Could you check a few things on this model? Use its own coordinates, in mm. A direction names the side the tool comes from. Give positions to 0.01 mm unless a question says otherwise; leave off trailing zeros. Write each loop counter-clockwise with the first axis right and the second up, starting at its lowest first coordinate (ties: lowest second). Pieces come first, ordered by that corner, then holes. Notation, with made-up numbers: M 26.25,23 L 69.25,23 A16 ccw 69.25,41 Z; hole C -26.75,55 d1. An arc over 180 degrees is marked long. Answer as CSV lines item,"result". Start each with the question number.
from build123d import *

# Parameters (mm, degrees)
F0_R     = 1.55
F1_DEPTH = 6


with BuildPart() as f1:
    # F0 (on Top) → F1 (new body)
    with BuildSketch(Plane.XY):
        Polygon((-284.438, 0), (0, 0), (0, 40.6), (-6, 40.6), (-6, 55.6), (0, 55.6), (0, 100.6), (-6, 100.6), (-6, 115.6), (0, 115.6), (0, 156.2), (-284.438, 156.2), (-284.438, 115.6), (-278.438, 115.6), (-278.438, 100.6), (-284.438, 100.6), (-284.438, 55.6), (-278.438, 55.6), (-278.438, 40.6), (-284.438, 40.6), align=None)
        with Locations((-258.438, 33.1)):
            Circle(F0_R, mode=Mode.SUBTRACT)
        with Locations((-248.438, 33.1)):
            Circle(F0_R, mode=Mode.SUBTRACT)
        with Locations((-258.438, 63.1)):
            Circle(F0_R, mode=Mode.SUBTRACT)
        with Locations((-248.438, 63.1)):
            Circle(F0_R, mode=Mode.SUBTRACT)
        with Locations((-36, 33.1)):
            Circle(F0_R, mode=Mode.SUBTRACT)
        with Locations((-26, 33.1)):
            Circle(F0_R, mode=Mode.SUBTRACT)
        with Locations((-36, 63.1)):
            Circle(F0_R, mode=Mode.SUBTRACT)
        with Locations((-26, 63.1)):
            Circle(F0_R, mode=Mode.SUBTRACT)
        with Locations((-258.438, 93.1)):
            Circle(F0_R, mode=Mode.SUBTRACT)
        with Locations((-248.438, 93.1)):
            Circle(F0_R, mode=Mode.SUBTRACT)
        with Locations((-258.438, 123.1)):
            Circle(F0_R, mode=Mode.SUBTRACT)
        with Locations((-248.438, 123.1)):
            Circle(F0_R, mode=Mode.SUBTRACT)
        with Locations((-36, 93.1)):
            Circle(F0_R, mode=Mode.SUBTRACT)
        with Locations((-26, 93.1)):
            Circle(F0_R, mode=Mode.SUBTRACT)
        with Locations((-36, 123.1)):
            Circle(F0_R, mode=Mode.SUBTRACT)
        with Locations((-26, 123.1)):
            Circle(F0_R, mode=Mode.SUBTRACT)
    extrude(amount=F1_DEPTH)


solid = f1.part
1. Thinking about a two-plate mould opening in Z: for faces 4 (the flat face through (-144, 79, 0)), 5 (the flat face through (-284.438, 78, 3)), which applies, pulls with the +Z half, pulls with the -Z half, needs draft (parallel to the pull), parting line crosses it, or undercut?
2. On a 3-axis mill with a long thin cutter (end or side, diameter ignored), from which of +Z, -Z, +X, -X, +Y, -Y can I reach the whole of each face in a straight line? I mean faces 1 (the flat face through (-3, 55.6, 3)), 2 (the flat face through (-284.438, 136, 3)), 3 (the flat face through (-278.438, 108, 3)). Say none if no direction works.
3. Please list where these lines run through material, in increasing order: line 1 (Y direction, x = -26, z = 1.45); line 2 (X direction, y = 123.1, z = 3.5); line 3 (X direction, y = 101, z = 1.25).
4. Imagine slicing it at A-A, the plane y = 44. Please give me the cut outline in (x, z).
5. Will these pins go through, and if not, where does the flat tip stop? P1, Ø3, axis at y = 48.5, z = 1.5, coming from the +X side; P2, Ø3, axis at y = 50.5, z = 3, coming from the -X side.
Solutions:
1,face 4,"pulls with the -Z half"
1,face 5,"needs draft"
2,face 1,"+Z, -Z, +X"
2,face 2,"+Z, -Z, -X, +Y, -Y"
2,face 3,"+Z, -Z, -X"
3,line 1,"0 to 31.55, 34.65 to 61.55, 64.65 to 91.55, 94.65 to 121.55, 124.65 to 156.2"
3,line 2,"-284.44 to -259.99, -256.89 to -249.99, -246.89 to -37.55, -34.45 to -27.55, -24.45 to 0"
3,line 3,"-278.44 to -6"
4,outline,"M -278.44,0 L -6,0 L -6,6 L -278.44,6 Z"
5,P1,"x = -6"
5,P2,"x = -278.44"
